Part model, mm, in its own coordinate system. Face numbers are marked on the shaded views. A direction names the side the tool comes from. Coordinates: 2 decimals unless noted, no trailing zeros. Write each loop counter-clockwise with the first axis right and the second up, starting at its lowest first coordinate (ties: lowest second). Pieces come first, ordered by that corner, then holes. Notation, with made-up numbers: (25, 5) -> (57, 5) arc R30 ccw to (57, 44) -> close; hole circle Ø1 at (50.5, -17). An arc over 180 degrees is marked (long way). Write item = value, one per line. Start each with the question number.
Q1. Probe line 1 (Y direction, x = -12, z = 2); line 2 (X direction, y = -52, z = 1.9); line 3 (Y direction, x = 1.5, z = 3.65). List the from-to ranges inside material, lowest first.
Q2. Pull direction X, two halves, no side cores. Call the marked faces 1, 2 and 3: released by +X, released by -X, zero draft, split by the parting line, or undercut.
Q3. Band-saw the part on C-C, the plane y = -2. List the corners of the cut face in (x, z), plus the area to 3 significant figures.
Q4. Band-saw the part on A-A, the plane y = -16. List the corners of the cut face in (x, z), plus the area to 3 significant figures.
Q5. Band-saw the part on B-B, the plane x = -11.75. List the corners of the cut face in (y, z), plus the area to 3 significant figures.
Q6. Tool access for the marked faces 4, 5 and 6: list every direction of +Z, -Z, +X, -X, +Y, -Y with a clear straight run to the whole face (end or side of a thin tool).
Q7. Pin check, flat tips, straight feed: P1, Ø2, axis at y = -2, z = 1.5, coming from the -X side; P2, Ø1.2, axis at y = -2.5, z = 1.5, coming from the +X side. Stop position of each tip, or through.
Q8. Band-saw the part on D-D, the plane z = 2.1. Give the number of separate pieces and of enclosed holes in the cut face, plus the area to 3 significant figures.
Autodesk Inventor part; units mm, degrees
ref_plane "YZ Plane" through (0, 0, 0) normal (1, 0, 0) x (0, 1, 0)
ref_plane "XZ Plane" through (0, 0, 0) normal (0, 1, 0) x (-1, 0, 0)
ref_plane "XY Plane" through (0, 0, 0) normal (0, 0, 1) x (1, 0, 0)
sketch "Sketch1" plane through (0, 0, 0) normal (0, 0, 1) x (1, 0, 0)
  line L0 (-15, 0) -> (15, 0)
  line L1 (15, 0) -> (15, -60)
  line L2 (15, -60) -> (-15, -60)
  line L3 (-15, -60) -> (-15, 0)
  line L4 (-21, 0) -> (21, 0)
  line L5 (0, -72) -> (0, 12)
  point P0 (0, 0)
  dimension "d0" = 30
  dimension "d1" = 60
  dimension "d4" = 15
extrude "Extrusion1" add sketch "Sketch1" along normal blind 4
sketch "Sketch2" plane through (0, 0, 4) normal (0, 0, 1) x (1, 0, 0)
  line L0 (15, 0) -> (-15, 0)
  line L1 (-15, 0) -> (-15, -60)
  line L2 (-15, -60) -> (15, -60)
  line L3 (15, -60) -> (15, 0)
  line L4 (0, -72) -> (0, 12)
  circle A0 centre (-12, -21) radius 1.5
  circle A1 centre (-12, -45) radius 1.5
  circle A2 centre (12, -21) radius 1.5
  circle A3 centre (12, -45) radius 1.5
  line L5 (15, 0) -> (-15, 0)
  line L6 (15, -60) -> (15, 0)
  line L7 (4.7021, 0) -> (15, 0)
  line L8 (15, 0) -> (15, -4)
  line L9 (15, -4) -> (4.7021, -4)
  line L10 (4.7021, -4) -> (4.7021, 0)
  line L11 (-15, 0) -> (-15, -60)
  line L12 (-5.2979, 0) -> (-15, 0)
  line L13 (-15, 0) -> (-15, -4)
  line L14 (-15, -4) -> (-5.2979, -4)
  line L15 (-5.2979, -4) -> (-5.2979, 0)
  line L16 (-3, -9) -> (3, -9)
  line L17 (5, -11) -> (5, -53)
  line L18 (3, -55) -> (-3, -55)
  line L19 (-5, -53) -> (-5, -11)
  arc A4 (-3, -9) -> (-5, -11) centre (-3, -11) ccw
  arc A5 (5, -11) -> (3, -9) centre (3, -11) ccw
  arc A6 (3, -55) -> (5, -53) centre (3, -53) ccw
  arc A7 (-5, -53) -> (-3, -55) centre (-3, -53) ccw
  point P0 (0, 0)
  dimension "d5" = 3
  dimension "d6" = 12
  dimension "d7" = 3
  dimension "d8" = 12
  dimension "d9" = 24
  dimension "d10" = 15
  dimension "d13" = 4
  dimension "d14" = 10
  dimension "d15" = 5
  dimension "d16" = 10
  dimension "d18" = 5
  dimension "d19" = 2
  dimension "d28" = 10
extrude "Extrusion2" cut sketch "Sketch2" against normal blind 4 contours L3 L9 L10 L0 | L15 L14 L1 L0 | L16 A5 L17 A6 L18 L4 | L4 L18 A7 L19 A4 L16 | A0 | A1 | A2 | A3
sketch "Sketch3" plane through (0, 0, 4) normal (0, 0, 1) x (1, 0, 0)
  point P0 (0, 0)
fillet "Fillet1" radius 2 2 edges at (15, -60, 2) (-15, -60, 2)
sketch "Sketch4" plane through (4.7021, -4, 4) normal (1, 0, 0) x (0, 0, -1)
  line L0 (0, 0) -> (0, 4)
  line L1 (0, 0) -> (4, 0)
  line L2 (4, 4) -> (4, 0)
  line L3 (0, 4) -> (4, 4)
  line L4 (0, 0) -> (4, 0)
  line L5 (2, 0) -> (2, 4) construction
  line L6 (0, 4) -> (4, 4)
  circle A0 centre (2, 2) radius 1
  dimension "d21" = 2
extrude "Extrusion3" cut sketch "Sketch4" against normal through all contours A0
sketch "Sketch5" plane through (15, -4, 4) normal (1, 0, 0) x (0, 0, -1)
  line L0 (4, -54) -> (0, -54)
  line L1 (4, 0) -> (4, -54)
  line L2 (4, 0) -> (0, 0)
  line L3 (0, -54) -> (0, 0)
  circle A0 centre (2, 2) radius 1
  circle A1 centre (2, 2) radius 1
  line L4 (2, 2) -> (2, -25.9382) construction
  circle A2 centre (2, -12) radius 1
  point P0 (4, 4)
  dimension "d24" = 2
  dimension "d25" = 14
extrude "Extrusion4" cut sketch "Sketch5" against normal through all contours A2
equation "\"d4\" = 0.5 * d0"
properties part number "BallBalancing_MotorPlate"
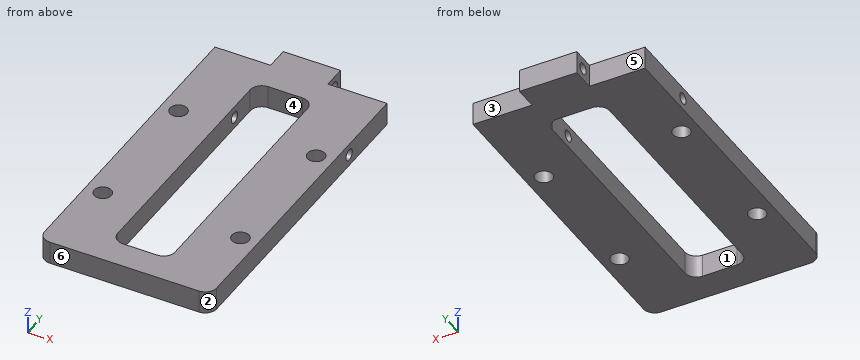
Ans:
q1.line_1 = -60 to -46.5, -43.5 to -22.5, -19.5 to -17, -15 to -4
q1.line_2 = -15 to -5, 5 to 15
q1.line_3 = -60 to -55, -9 to 0
q2.face_1 = undercut
q2.face_2 = released by +X
q2.face_3 = zero draft
q3.outline = (-5.3, 0) -> (4.7, 0) -> (4.7, 1) -> (-5.3, 1) -> close; (-5.3, 3) -> (4.7, 3) -> (4.7, 4) -> (-5.3, 4) -> close
q3.area = 20.0 mm2
q4.outline = (-15, 0) -> (-5, 0) -> (-5, 1) -> (-15, 1) -> close; (-15, 3) -> (-5, 3) -> (-5, 4) -> (-15, 4) -> close; (5, 0) -> (15, 0) -> (15, 1) -> (5, 1) -> close; (5, 3) -> (15, 3) -> (15, 4) -> (5, 4) -> close
q4.area = 40.0 mm2
q5.outline = (-60, 0) -> (-46.48, 0) -> (-46.48, 4) -> (-60, 4) -> close; (-43.52, 0) -> (-22.48, 0) -> (-22.48, 4) -> (-43.52, 4) -> close; (-19.52, 0) -> (-4, 0) -> (-4, 4) -> (-19.52, 4) -> close; hole circle Ø2 at (-16, 2)
q5.area = 197 mm2
q6.face_4 = +Z, -Z
q6.face_5 = +Z, -Z, -X, +Y
q6.face_6 = +Z, -Z, +X, -X, -Y
q7.P1 = -5.3
q7.P2 = 4.7
q8.separate_pieces = 3
q8.enclosed_holes = 4
q8.area = 1,170 mm2
